from build123d import *

# Parameters (mm, degrees)
SKETCH092_R             = 6
PAD066_DEPTH            = 3
SKETCH093_W             = 26
SKETCH093_H             = 4
PAD067_DEPTH            = 30
SKETCH094_R             = 2
POCKET034_DEPTH         = 31.001
SKETCH095_R             = 1
POCKET035_DEPTH         = 137.42322
POLARPATTERN014_COUNT   = 4
BODY040_PLACEMENT_ANGLE = 215


with BuildPart() as part:
    # Sketch092 → Pad066 (new body)
    with BuildSketch(Plane.XZ):
        with BuildLine():
            Line((-13, 18), (13, 18))
            Line((13, 18), (13, 0))
            ThreePointArc((-13, 0), (0, -13), (13, 0))
            Line((-13, 18), (-13, 0))
        make_face()
        Circle(SKETCH092_R, mode=Mode.SUBTRACT)
    extrude(amount=PAD066_DEPTH)

    # Sketch093 (on Face7 of Pad066) → Pad067 (join)
    with BuildSketch(Plane.XZ.offset(3)):
        with Locations((0, 16)):
            Rectangle(SKETCH093_W, SKETCH093_H)
    extrude(amount=PAD067_DEPTH)

    # Sketch094 (on Face5 of Pad067) → Pocket034 (cut, through all)
    with BuildSketch(Plane(origin=(0, 0, 18), x_dir=(-1, 0, 0), z_dir=(0, 0, 1))):
        with Locations((-9, 7)):
            Circle(SKETCH094_R)
        with Locations((9, 7)):
            Circle(SKETCH094_R)
        with Locations((-9, 29)):
            Circle(SKETCH094_R)
        with Locations((9, 29)):
            Circle(SKETCH094_R)
    extrude(amount=-POCKET034_DEPTH, mode=Mode.SUBTRACT)

    # Sketch095 (on Face4 of Pocket034) → Pocket035 (cut, through all)
    with BuildSketch(Plane(origin=(0, 0, 0), x_dir=(1, 0, 0), z_dir=(0, 1, 0))):
        with Locations((0, 9.5)):
            Circle(SKETCH095_R)
    pocket035 = extrude(amount=-POCKET035_DEPTH, mode=Mode.SUBTRACT)

    # PolarPattern014: Pocket035 ×4 about axis
    polarpattern014_axis = Axis((0, 0, 0), (0, 1, 0))
    for i in range(1, POLARPATTERN014_COUNT):
        add(pocket035.rotate(polarpattern014_axis, i * 360 / POLARPATTERN014_COUNT), mode=Mode.SUBTRACT)


with BuildPart() as part_1:
    # Body040 placement: moved
    add(part.part.moved(Location((43.591809, -62.255555, -8))).rotate(Axis((43.591809, -62.255555, -8), (0, 0, 1)), BODY040_PLACEMENT_ANGLE))


solid = part_1.part
Design review of the part built by this model. Coordinates are the model's own, in mm. A direction names the side the tool comes from. Round coordinates to 2 decimals unless told otherwise and drop trailing zeros. Order: outer loops, then holes, each group sorted by start corner. A loop starts at its lowest first (then second) coordinate and runs counter-clockwise, first axis right, second up.
1) Consider section D-D (y = -36). State the section outline as (x, z) points.
The answers:
outline: (23.55, 6) - (41.08, 6) - (41.08, 10) - (23.55, 10) - close
2) Consider section B-B (z = -3.5). State the section outline as (x, y) points, plus the area to 3 significant figures.
The answers:
outline: (31.22, -67.25) - (32.94, -69.71) - (40.34, -64.53) - (38.62, -62.07) - close; (45.12, -57.52) - (46.84, -59.98) - (54.24, -54.8) - (52.52, -52.34) - close
area: 54.2 mm2
3) For L1, parallel to Z at x = 26, y = -43; L2, parallel to X at y = -51.5, z = 7; L3, parallel to Y at x = 51, z = -6, list the stretches that pass through material, from the lowest coordinate up.
The answers:
L1: z = 6 to 10
L2: x = 20.19 to 44.95, 48.94 to 51.93
L3: y = -57.07 to -53.41
4) Machinability: for faces 5 (the flat face through (41.722, -59.902, -1.311)), 6 (the cylindrical face through (42.37, -61.31, -16.61)), which of the approach directions +Z, -Z, +X, -X, +Y, -Y give a long, thin tool a straight path to every point of the face, cutting with its end or side? Answer none if there is none.
The answers:
face 5: -Z, -X, +Y
face 6: none
5) Draft analysis for pull direction X (two halves, no side actions). For faces 1 (the cylindrical face through (32.64, -34.41, 8.03)), 2 (the flat face through (47.625, -45.351, 6.291)), 3 (the flat face through (34, -49, 10)), 4 (the flat face through (26.327, -60.264, 6.291)), state which applies: released by +X, released by -X, zero draft, split by the parting line, or undercut.
The answers:
face 1: undercut
face 2: released by +X
face 3: zero draft
face 4: released by -X
6) Consider section A-A (z = 7.5). State the section outline as (x, y) points, plus the area to 3 significant figures.
The answers:
outline: (14.01, -42.68) - (32.94, -69.71) - (54.24, -54.8) - (35.31, -27.77) - close; hole circle Ø4 at (19.59, -43.66); hole circle Ø4 at (32.2, -61.68); hole circle Ø4 at (34.33, -33.34); hole circle Ø4 at (46.95, -51.36)
area: 808 mm2
7) Clearance check with flat-ended pins moving along their axes: pin 1 Ø6 at (y, z) = (-51, -8.5) entering from -X; pin 2 Ø5 at (x, y) = (34.33, -33.34) entering from -Z; pin 3 Ø5 at (x, y) = (50, -59.5) entering from -Z; pin 4 Ø19.5 at (x, y) = (36.5, -52.5) entering from -Z. State where each tip first meets the part, or that it passes through.
The answers:
pin 1: stops at x = 50.17
pin 2: stops at z = 6
pin 3: stops at z = -20.09
pin 4: stops at z = -21
8) Consider section C-C (x = 45.5). Count the separate pieces of the cut face and the enclosed holes in it, plus the area to 3 significant figures.
The answers:
separate pieces: 3
enclosed holes: 0
area: 125 mm2
